```python
from build123d import *

# Parameters (mm, degrees)
F0_R     = 25
F1_DEPTH = 5
F2_R     = 17.5
F3_DEPTH = 105
F4_R     = 15.5
F5_DEPTH = 105
F6_R     = 2.49999
F7_R     = 3.8034251557
F8_DEPTH = 30


# Not quite as in the source:
# - a fillet or chamfer is up to 0.001 mm smaller than in the source, because OpenCascade refuses the exact size


with BuildPart() as f1:
    # F0 (on Top) → F1 (new body)
    with BuildSketch(Plane.XY):
        Circle(F0_R)
    extrude(amount=F1_DEPTH)

    # F2 (on face) → F3 (join)
    with BuildSketch(Plane.XY.offset(5)):
        Circle(F2_R)
    extrude(amount=F3_DEPTH)

    # F4 (on face) → F5 (cut)
    with BuildSketch(Plane(origin=(0, 0, 0), x_dir=(1, 0, 0), z_dir=(0, 0, -1))):
        Circle(F4_R)
    extrude(amount=-F5_DEPTH, mode=Mode.SUBTRACT)

    # F6 (radius 2.5 in the source; OpenCascade refuses exactly that, so slightly less here)
    f6_edges = [f1.edges().sort_by_distance(p)[0] for p in [
        (-17.5, 0, 110),
        (-17.5, 0, 5),
        (-25, 0, 5),
        (-25, 0, 0),
    ]]
    fillet(f6_edges, radius=F6_R)

    # F7 (on face) → F8 (cut)
    with BuildSketch(Plane.XY.offset(110)):
        Circle(F7_R)
    extrude(amount=-F8_DEPTH, mode=Mode.SUBTRACT)


solid = f1.part
```
Design review of the part built by this model. Coordinates are the model's own, in mm. A direction names the side the tool comes from. Give positions to 0.01 mm unless a question says otherwise; leave off trailing zeros. Loops run counter-clockwise (first coordinate to the right, second up) from the corner with the lowest first, then second, coordinate; pieces in that order, holes last. Notation, with made-up numbers: (-27, 68.5) -> (17, 68.5) arc R15 cw to (17, 87.5) -> close; hole circle Ø2 at (15, 67.5). An arc over 180 degrees is marked (long way). One line per item, written item: value.
Q1. For L1, parallel to Y at x = 0, z = 70.5; L2, parallel to X at y = 0.5, z = 55; L3, parallel to Y at x = 0, z = 106, list the stretches that pass through material, from the lowest coordinate up.
Numbers:
L1: y = -17.5 to -15.5, 15.5 to 17.5
L2: x = -17.49 to -15.49, 15.49 to 17.49
L3: y = -17.5 to -3.8, 3.8 to 17.5
Q2. Machinability: for faces 4 (the cylindrical face through (-0.5, 3.77, 107.54)), 5 (the cylindrical face through (-2.018, -15.368, 51.765)), which of the approach directions +Z, -Z, +X, -X, +Y, -Y give a long, thin tool a straight path to every point of the face, cutting with its end or side? Answer none if there is none.
Numbers:
face 4: +Z, -Z
face 5: -Z
Q3. We need section C-C on z = 82. Give the boundary of the cut face in (x, y), and give its area (3 significant figures).
Numbers:
outline: circle Ø35 at (0, 0); hole circle Ø31 at (0, 0)
area: 207 mm^2
Q4. Draft analysis for pull direction X (two halves, no side actions). For faces 1 (the flat face through (3, 3, 105)), 2 (the cylindrical face through (-13.887, -10.648, 56.8)), 3 (the flat face through (-20.1, -1.6, 5)), state which applies: pulls with the +X half, pulls with the -X half, needs draft (parallel to the pull), parting line crosses it, or undercut.
Numbers:
face 1: undercut
face 2: parting line crosses it
face 3: needs draft
Q5. For pin 1 Ø10 at (y, z) = (8, 68.5) entering from +X; pin 2 Ø6 at (x, z) = (-19, 74.5) entering from +Y; pin 3 Ø2 at (y, z) = (-10.5, 50.5) entering from +X, all flat-tipped, find the tip position at first contact; note any pin that passes through.
Numbers:
pin 1: stops at x = 17.24
pin 2: stops at y = 7.09
pin 3: stops at x = 14.7
